```python
from build123d import *

# Parameters (mm, degrees)
SCHIZZO1_W                   = 450
SCHIZZO1_H                   = 160
ESTRUSIONE_ESTRUSIONE1_DEPTH = 10
SCHIZZO2_R                   = 12.5
SCHIZZO2_R_2                 = 2.25
TAGLIO_ESTRUSIONE1_DEPTH     = 10


with BuildPart() as part:
    # Schizzo1 → Estrusione-Estrusione1 (new body)
    with BuildSketch(Plane.XY):
        with Locations((225, 80)):
            Rectangle(SCHIZZO1_W, SCHIZZO1_H)
    extrude(amount=ESTRUSIONE_ESTRUSIONE1_DEPTH)

    # Schizzo2 → Taglio-Estrusione1 (cut)
    with BuildSketch(Plane.XY.offset(10)):
        with Locations((347.5, 36)):
            Circle(SCHIZZO2_R)
        with Locations((382, 154.5)):
            Circle(SCHIZZO2_R_2)
        with Locations((382, 136)):
            Circle(SCHIZZO2_R_2)
        with Locations((68, 154.5)):
            Circle(SCHIZZO2_R_2)
        with Locations((68, 136)):
            Circle(SCHIZZO2_R_2)
        with Locations((38, 42)):
            Circle(SCHIZZO2_R_2)
        with Locations((38, 23.5)):
            Circle(SCHIZZO2_R_2)
        with Locations((422, 23.5)):
            Circle(SCHIZZO2_R_2)
        with Locations((422, 42)):
            Circle(SCHIZZO2_R_2)
        with Locations((23.5, 134.933694222)):
            Circle(SCHIZZO2_R_2)
        with Locations((42, 134.933694222)):
            Circle(SCHIZZO2_R_2)
        with Locations((28, 70)):
            Circle(SCHIZZO2_R_2)
        with Locations((422, 85)):
            Circle(SCHIZZO2_R_2)
        with Locations((312.5, 95)):
            Circle(SCHIZZO2_R_2)
        with Locations((382.5, 95)):
            Circle(SCHIZZO2_R_2)
        with Locations((382.5, 35)):
            Circle(SCHIZZO2_R_2)
        with Locations((312.5, 35)):
            Circle(SCHIZZO2_R_2)
        with BuildLine():
            Line((87.5, 42), (117.5, 42))
            ThreePointArc((117.5, 42), (123.5, 36), (117.5, 30))
            Line((117.5, 30), (87.5, 30))
            ThreePointArc((87.5, 30), (81.5, 36), (87.5, 42))
        make_face()
    extrude(amount=-TAGLIO_ESTRUSIONE1_DEPTH, mode=Mode.SUBTRACT)


solid = part.part
```
The listing builds one solid part. Answer for the finished solid, in the listing's coordinates (mm). A direction names the side the tool comes from. Round coordinates to 2 decimals unless told otherwise and drop trailing zeros. Order: outer loops, then holes, each group sorted by start corner. A loop starts at its lowest first (then second) coordinate and runs counter-clockwise, first axis right, second up. Notation, with made-up numbers: (44.25, 24) -> (56.25, 24) arc R22 cw to (56.25, 54) -> close; hole circle Ø4 at (85.25, 46.25). An arc over 180 degrees is marked (long way). Answer as CSV lines item,"result".
Q1. Consider line 1 (Y direction, x = 382.5, z = 4.5); line 2 (Y direction, x = 38, z = 4.5); line 3 (Y direction, x = 422, z = 6.5). Determine where each line is inside the solid, lowest interval first. Write a range as from..to.
Computed values:
line 1,"y = 0..32.75, 37.25..92.75, 97.25..133.81, 138.19..152.31, 156.69..160"
line 2,"y = 0..21.25, 25.75..39.75, 44.25..160"
line 3,"y = 0..21.25, 25.75..39.75, 44.25..82.75, 87.25..160"
Q2. A cutting plane is placed at A-A on x = 347.5. Determine the outline of the cut face in (y, z).
Computed values:
outline,"(0, 0) -> (23.5, 0) -> (23.5, 10) -> (0, 10) -> close; (48.5, 0) -> (160, 0) -> (160, 10) -> (48.5, 10) -> close"
Q3. A cutting plane is placed at B-B on z = 1.5. Give the number of separate pieces and of enclosed holes in the cut face, plus the area to 3 significant figures.
Computed values:
separate pieces,"1"
enclosed holes,"18"
area,"70,800 mm^2"
Q4. Which of the six approach directions +Z, -Z, +X, -X, +Y, -Y give full straight-line access (tool end or side, diameter ignored) to faces 4 (the flat face through (103, 30, 5)), 5 (the flat face through (222, 0, 5))?
Computed values:
face 4,"+Z, -Z"
face 5,"+Z, -Z, +X, -X, -Y"
Q5. For a pull along X with two mould halves and no side action, classify faces 1 (the flat face through (222, 81, 0)), 2 (the cylindrical face through (359.423, 39.755, 5.07)), 3 (the flat face through (0, 79, 5)) as +X half, -X half, draft (parallel to the pull), parting line (faces both ways), or undercut.
Computed values:
face 1,"draft"
face 2,"undercut"
face 3,"-X half"
